Input: part model. Units: mm. Frame: model coordinates. Face numbers are marked on the shaded views. Coordinates: 2 decimals unless noted, no trailing zeros. Order: outer loops, then holes, each group sorted by start corner. A loop starts at its lowest first (then second) coordinate and runs counter-clockwise, first axis right, second up. Notation, with made-up numbers: (35.5, -39) - (47.5, -39) arc R25 ccw to (47.5, -24) - close; hole circle Ø10 at (8.25, 46). An arc over 180 degrees is marked (long way). One line per question, with ' | ' between items.
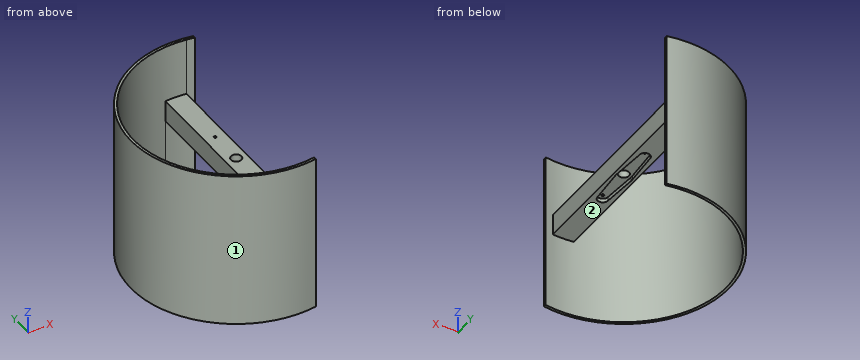
from build123d import *

# Parameters (mm, degrees)
ESQUISSE1_W              = 8
ESQUISSE1_H              = 79
BOSS_EXTRU_1_DEPTH       = 60
ESQUISSE3_R              = 40
ESQUISSE3_R_2            = 39
BOSS_EXTRU_2_DEPTH       = 60
ESQUISSE4_R              = 39
ENL_V_MAT_EXTRU_3_DEPTH  = 30
ENL_V_MAT_EXTRU_5_DEPTH  = 1.5
ESQUISSE6_R              = 39
ENL_V_MAT_EXTRU_6_DEPTH  = 22
ESQUISSE7_R              = 2
ENL_V_MAT_EXTRU_7_DEPTH  = 6.5
ESQUISSE9_R              = 0.5
ENL_V_MAT_EXTRU_8_DEPTH  = 29.5
ENL_V_MAT_EXTRU_10_REACH = 62
ESQUISSE11_W             = 40
ESQUISSE11_H             = 82


with BuildPart() as part:
    # Esquisse1 → Boss.-Extru.1 (new body)
    with BuildSketch(Plane.XY):
        with Locations((4, 39.5)):
            Rectangle(ESQUISSE1_W, ESQUISSE1_H)
    extrude(amount=BOSS_EXTRU_1_DEPTH)

    # Esquisse3 → Boss.-Extru.2 (add)
    with BuildSketch(Plane(origin=(0, 0, 0), x_dir=(-1, 0, 0), z_dir=(0, 0, -1))):
        with Locations((-4, 39.5)):
            Circle(ESQUISSE3_R)
        with Locations((-4, 39.5)):
            Circle(ESQUISSE3_R_2, mode=Mode.SUBTRACT)
    extrude(amount=-BOSS_EXTRU_2_DEPTH)

    # Esquisse4 → Enlèv. mat.-Extru.3 (cut)
    with BuildSketch(Plane(origin=(0, 0, 0), x_dir=(-1, 0, 0), z_dir=(0, 0, -1))):
        with Locations((-4, 39.5)):
            Circle(ESQUISSE4_R)
    extrude(amount=-ENL_V_MAT_EXTRU_3_DEPTH, mode=Mode.SUBTRACT)

    # Esquisse5 → Enlèv. mat.-Extru.5 (cut)
    with BuildSketch(Plane(origin=(0, 0, 30), x_dir=(-1, 0, 0), z_dir=(0, 0, -1))):
        with BuildLine():
            Line((-6, 53), (-6.967257844, 39.9420191))
            ThreePointArc((-6.967257844, 39.9420191), (-7, 39.5), (-6.967257844, 39.0579809))
            Line((-6.967257844, 39.0579809), (-6, 26))
            ThreePointArc((-6, 26), (-4, 24), (-2, 26))
            Line((-2, 26), (-1.032742156, 39.0579809))
            ThreePointArc((-1.032742156, 39.0579809), (-1, 39.5), (-1.032742156, 39.9420191))
            Line((-1.032742156, 39.9420191), (-2, 53))
            ThreePointArc((-2, 53), (-4, 55), (-6, 53))
        make_face()
    extrude(amount=-ENL_V_MAT_EXTRU_5_DEPTH, mode=Mode.SUBTRACT)

    # Esquisse6 → Enlèv. mat.-Extru.6 (cut)
    with BuildSketch(Plane.XY.offset(60)):
        with Locations((4, 39.5)):
            Circle(ESQUISSE6_R)
    extrude(amount=-ENL_V_MAT_EXTRU_6_DEPTH, mode=Mode.SUBTRACT)

    # Esquisse7 → Enlèv. mat.-Extru.7 (cut)
    with BuildSketch(Plane(origin=(0, 0, 31.5), x_dir=(-1, 0, 0), z_dir=(0, 0, -1))):
        with Locations((-4, 39.5)):
            Circle(ESQUISSE7_R)
    extrude(amount=-ENL_V_MAT_EXTRU_7_DEPTH, mode=Mode.SUBTRACT)

    # Esquisse9 → Enlèv. mat.-Extru.8 (cut, through all)
    with BuildSketch(Plane(origin=(0, 0, 31.5), x_dir=(-1, 0, 0), z_dir=(0, 0, -1))):
        with Locations((-4, 53)):
            Circle(ESQUISSE9_R)
        with Locations((-4, 26)):
            Circle(ESQUISSE9_R)
    extrude(amount=-ENL_V_MAT_EXTRU_8_DEPTH, mode=Mode.SUBTRACT)

    # Esquisse11 → Enlèv. mat.-Extru.10 (cut, up to next)
    with BuildSketch(Plane.XY, mode=Mode.PRIVATE) as enl_v_mat_extru_10_sk1:
        with Locations((31, 39.5)):
            Rectangle(ESQUISSE11_W, ESQUISSE11_H)
    enl_v_mat_extru_10_tool1 = extrude(enl_v_mat_extru_10_sk1.sketch, amount=ENL_V_MAT_EXTRU_10_REACH, mode=Mode.PRIVATE) & part.part
    add(enl_v_mat_extru_10_tool1.solids().sort_by_distance((31, 39.5, 0))[0], mode=Mode.SUBTRACT)


solid = part.part
Item 1: Draft query along Y for the marked faces 1 and 2. Return one class per face: released by +Y, released by -Y, zero draft, split by the parting line, or undercut.
Data:
face 1: split by the parting line | face 2: undercut
Item 2: Section D-D on x = -23.5. Return the cut outline in (y, z).
Data:
outline: (10.45, 0) - (11.85, 0) - (11.85, 60) - (10.45, 60) - close; (67.15, 0) - (68.55, 0) - (68.55, 60) - (67.15, 60) - close
Item 3: Contact query for flat-ended pins moving along their axis: P1, Ø8, axis at x = -5, z = 30, coming from the +Y side; P2, Ø5, axis at x = -7.5, z = 10, coming from the -Y side; P3, Ø8, axis at y = 29.5, z = 17, coming from the -X side; P4, Ø2, axis at x = -20, y = 9.5, coming from the +Z side. Output: stop coordinate, or through.
Data:
P1: y = 79.19 | P2: y = 0.53 | P3: x = -35.55 | P4: z = 60
Item 4: Ray query, line 1 (Y direction, x = 4, z = 33.5); line 2 (X direction, y = 39, z = 36); line 3 (Z direction, x = 3.5, y = 69). Return the intervals inside material, ascending.
Data:
line 1: -0.5 to 25.5, 26.5 to 37.5, 41.5 to 52.5, 53.5 to 79.5 | line 2: -36 to -35, 0 to 2.06, 5.94 to 8 | line 3: 30 to 38
Item 5: Section A-A on z = 35. Return the cut outline in (x, y).
Data:
outline: (8, 0.71) - (8, 78.29) arc R39 cw to (11, 77.87) - (11, 78.88) arc R40 ccw (long way) to (11, 0.12) - (11, 1.13) arc R39 cw to start; hole (0, 0.71) - (0, 78.29) arc R39 ccw to start; hole circle Ø4 at (4, 39.5); hole circle Ø1 at (4, 26); hole circle Ø1 at (4, 53)
Item 6: Section C-C on y = 33. Return the cut outline in (x, z), and give its area (3 significant figures).
Data:
outline: (-35.47, 0) - (-34.45, 0) - (-34.45, 60) - (-35.47, 60) - close; (0, 30) - (1.48, 30) - (1.48, 31.5) - (6.52, 31.5) - (6.52, 30) - (8, 30) - (8, 38) - (0, 38) - close | area: 117 mm^2
Item 7: Section B-B on x = -13. Return the cut outline in (y, z), and give its area (3 significant figures).
Data:
outline: (3.29, 0) - (4.4, 0) - (4.4, 60) - (3.29, 60) - close; (74.6, 0) - (75.71, 0) - (75.71, 60) - (74.6, 60) - close | area: 133 mm^2
